```python
from build123d import *

# Parameters (mm, degrees)
F0_R     = 2.38125
F1_DEPTH = 25.4
F2_DEPTH = 25.4


with BuildPart() as f1:
    # F0 (on Top) → F1 (new body)
    with BuildSketch(Plane.XY):
        with BuildLine():
            ThreePointArc((0, 381), (-32.870019, 376.67258), (-63.5, 363.985226))
            Line((-63.5, 363.985226), (-63.5, 259.4))
            Line((-63.5, 259.4), (-127, 222.738258))
            Line((-127, 222.738258), (-127, 203.2))
            Line((-127, 203.2), (127, 203.2))
            Line((127, 203.2), (127, 222.738258))
            Line((127, 222.738258), (63.5, 259.4))
            Line((63.5, 259.4), (63.5, 363.985226))
            ThreePointArc((63.5, 363.985226), (32.870019, 376.67258), (0, 381))
        make_face()
        with Locations((-20.6375, 297.5)):
            Circle(F0_R, mode=Mode.SUBTRACT)
        with Locations((-20.6375, 361)):
            Circle(F0_R, mode=Mode.SUBTRACT)
        with Locations((20.6375, 297.5)):
            Circle(F0_R, mode=Mode.SUBTRACT)
        with Locations((20.6375, 361)):
            Circle(F0_R, mode=Mode.SUBTRACT)
        with BuildLine():
            Line((0, 381), (-63.5, 381))
            Line((-63.5, 381), (-63.5, 363.985226))
            ThreePointArc((-63.5, 363.985226), (-32.870019, 376.67258), (0, 381))
        make_face()
        with BuildLine():
            Line((63.5, 381), (0, 381))
            ThreePointArc((0, 381), (32.870019, 376.67258), (63.5, 363.985226))
            Line((63.5, 363.985226), (63.5, 381))
        make_face()
    extrude(amount=F1_DEPTH)

    # F0 (on Top) → F2 (join)
    with BuildSketch(Plane.XY):
        with BuildLine():
            ThreePointArc((127, 254), (109.985226, 317.5), (63.5, 363.985226))
            Line((63.5, 363.985226), (63.5, 259.4))
            Line((63.5, 259.4), (127, 222.738258))
            Line((127, 222.738258), (127, 254))
        make_face()
        with BuildLine():
            ThreePointArc((0, 381), (-32.870019, 376.67258), (-63.5, 363.985226))
            Line((-63.5, 363.985226), (-63.5, 259.4))
            Line((-63.5, 259.4), (-127, 222.738258))
            Line((-127, 222.738258), (-127, 203.2))
            Line((-127, 203.2), (127, 203.2))
            Line((127, 203.2), (127, 222.738258))
            Line((127, 222.738258), (63.5, 259.4))
            Line((63.5, 259.4), (63.5, 363.985226))
            ThreePointArc((63.5, 363.985226), (32.870019, 376.67258), (0, 381))
        make_face()
        with Locations((-20.6375, 297.5)):
            Circle(F0_R, mode=Mode.SUBTRACT)
        with Locations((-20.6375, 361)):
            Circle(F0_R, mode=Mode.SUBTRACT)
        with Locations((20.6375, 297.5)):
            Circle(F0_R, mode=Mode.SUBTRACT)
        with Locations((20.6375, 361)):
            Circle(F0_R, mode=Mode.SUBTRACT)
        with BuildLine():
            Line((-63.5, 259.4), (-63.5, 363.985226))
            ThreePointArc((-63.5, 363.985226), (-109.985226, 317.5), (-127, 254))
            Line((-127, 254), (-127, 222.738258))
            Line((-127, 222.738258), (-63.5, 259.4))
        make_face()
    extrude(amount=-F2_DEPTH)


solid = f1.part
```
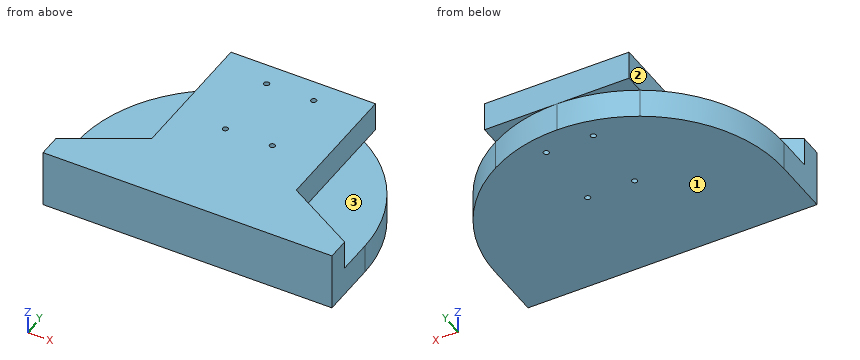
Can you work these out from the model? Positions are in its coordinate system, mm. Face numbers are marked on the shaded views. A direction names the side the tool comes from. Coordinates: 2 decimals unless noted, no trailing zeros. Loops run counter-clockwise (first coordinate to the right, second up) from the corner with the lowest first, then second, coordinate; pieces in that order, holes last. Notation, with made-up numbers: (-35.5, 49) - (10.5, 49) arc R11 ccw to (10.5, 70) - close; hole circle Ø4 at (42, -34). An arc over 180 degrees is marked (long way). Answer as CSV lines item,"result". Start each with the question number.
1) I need wall thicknesses on line 1 (X direction, y = 361, z = 18.25); line 2 (Z direction, x = 78, y = 260.5); line 3 (Y direction, x = -81, z = -1). Which ranges of each line are inside material? Lowest first, please. Write a range as from..to.
2) Suppose I cut it at A-A (z = -18). Please give me the cut outline in (x, y), plus the area to 3 significant figures.
3) For pin 1 (3 mm diameter, centred on x = -96.5, y = 274.5, fed in from +Z); pin 2 (12 mm diameter, centred on y = 313, z = -18.5, fed in from -X); pin 3 (1 mm diameter, centred on x = -86, z = 20, fed in from +Y); pin 4 (4 mm diameter, centred on x = -20.64, y = 297.5, fed in from +Z), each with a flat end and sliding along its axis, tell me the tip position at first contact or that it passes through.
4) Suppose I cut it at B-B (z = 10). Please give me the cut outline in (x, y), plus the area to 3 significant figures.
5) Suppose I cut it at C-C (y = 263). Please give me the cut outline in (x, z).
6) Which directions (+Z, -Z, +X, -X, +Y, -Y) give clear straight access to the entire face, cutting with the end or side of a thin tool? Please do the marked faces 1, 2 and 3.
7) Suppose I cut it at D-D (x = 53.5). Please give me the cut outline in (y, z).
Check result:
1,line 1,"x = -63.5..-23.02, -18.26..18.26, 23.02..63.5"
1,line 2,"z = -25.4..0"
1,line 3,"y = 203.2..351.82"
2,outline,"(-127, 203.2) - (127, 203.2) - (127, 254) arc R127 ccw to (63.5, 363.99) arc R127 ccw to (0, 381) arc R127 ccw to (-63.5, 363.99) arc R127 ccw to (-127, 254) - close; hole circle Ø4.76 at (-20.64, 297.5); hole circle Ø4.76 at (-20.64, 361); hole circle Ø4.76 at (20.64, 297.5); hole circle Ø4.76 at (20.64, 361)"
2,area,"38,200 mm²"
3,pin 1,"stops at z = 0"
3,pin 2,"stops at x = -115.41"
3,pin 3,"stops at y = 246.7"
3,pin 4,"passes through"
4,outline,"(-127, 203.2) - (127, 203.2) - (127, 222.74) - (63.5, 259.4) - (63.5, 381) - (-63.5, 381) - (-63.5, 259.4) - (-127, 222.74) - close; hole circle Ø4.76 at (-20.64, 297.5); hole circle Ø4.76 at (-20.64, 361); hole circle Ø4.76 at (20.64, 297.5); hole circle Ø4.76 at (20.64, 361)"
4,area,"27,300 mm²"
5,outline,"(-126.68, -25.4) - (126.68, -25.4) - (126.68, 0) - (63.5, 0) - (63.5, 25.4) - (-63.5, 25.4) - (-63.5, 0) - (-126.68, 0) - close"
6,face 1,"-Z, +X, -X, +Y, -Y"
6,face 2,"+Z, -X, +Y"
6,face 3,"+Z, +X, +Y"
7,outline,"(203.2, -25.4) - (369.18, -25.4) - (369.18, 0) - (381, 0) - (381, 25.4) - (203.2, 25.4) - close"
